For this review, use the dimensioned drawing (mm, ordinates from the lowest corner) and the shaded views. Coordinates: 2 decimals unless noted, no trailing zeros. Loops run counter-clockwise (first coordinate to the right, second up) from the corner with the lowest first, then second, coordinate; pieces in that order, holes last. Notation, with made-up numbers: (82.5, 12.25) - (117.5, 12.25) arc R17 ccw to (117.5, 21.25) - close; hole circle Ø6 at (29.5, -4). An arc over 180 degrees is marked (long way). One line per item, written item: value. Start each with the question number.
1. Insertion check: P1, Ø1.5, axis at y = 11, z = 1, coming from the -X side; P2, Ø1.5, axis at y = 11, z = 2, coming from the +X side; P3, Ø1.5, axis at x = 12.5, z = 1, coming from the +Y side. Each pin has a flat end and moves straight along its axis. Give the tip position at first contact, or say it passes through.
2. We need section D-D, the plane x = 27.5. Give the boundary of the cut face in (y, z).
3. To check wall thickness, follow line 1 (Y direction, x = 13.5, z = 1.5) (1 decimal); line 2 (Y direction, x = 33, z = 1.6) (1 decimal); line 3 (Y direction, x = 17, z = 2.15) (1 decimal). State the ranges of each line that lie inside material, in increasing order.
4. Mouldability with a two-part tool opening along X and no side actions: class the marked faces 1, 2, 3 and 4 as +X half, -X half, draft (parallel to the pull), parting line (faces both ways), or undercut.
5. We need section C-C, the plane z = 1.8. Give the boundary of the cut face in (x, y) (1 decimal), then the cut area to 3 significant figures.
6. We need section A-A, the plane x = 14. Give the boundary of the cut face in (y, z).
7. We need section B-B, the plane y = 12. Give the boundary of the cut face in (x, z).
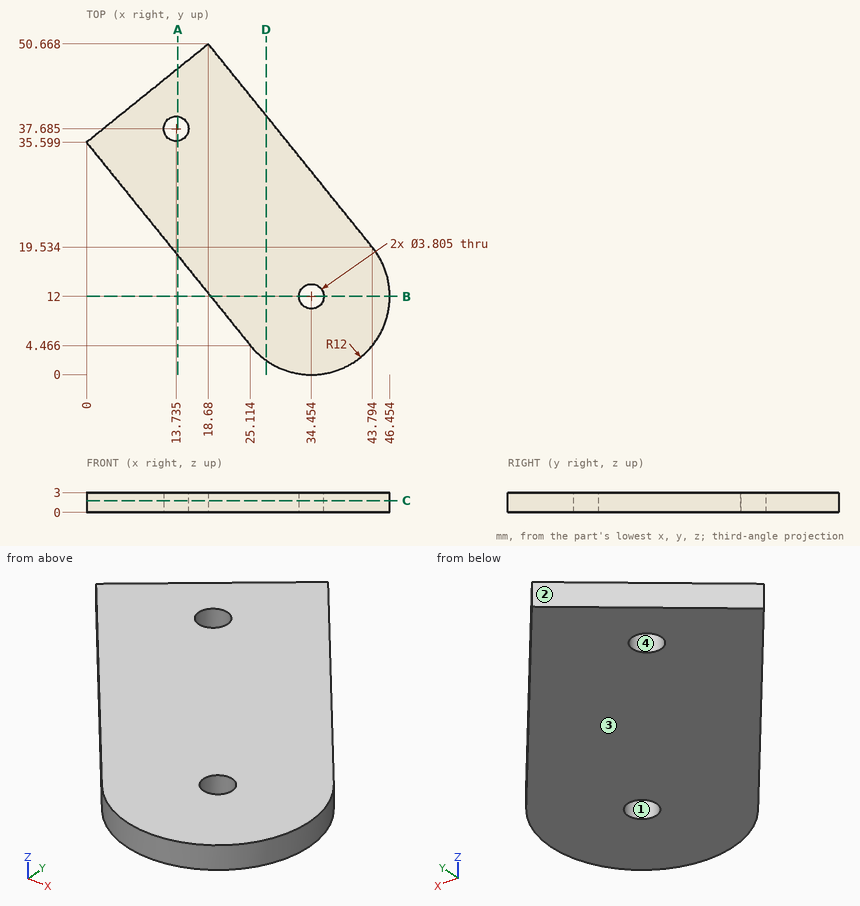
Findings below:
1. P1: x = 19.24
1. P2: x = 46.45
1. P3: y = 46.29
2. outline: (2.22, 0) - (39.73, 0) - (39.73, 3) - (2.22, 3) - close
3. line 1: 18.9 to 35.8, 39.6 to 46.5
3. line 2: 0.1 to 10.8, 13.2 to 32.9
3. line 3: 14.5 to 49.3
4. face 1: undercut
4. face 2: -X half
4. face 3: draft
4. face 4: undercut
5. outline: (0, 35.6) - (25.1, 4.5) arc R12 ccw to (43.8, 19.5) - (18.7, 50.7) - close; hole circle Ø3.8 at (13.7, 37.7); hole circle Ø3.8 at (34.5, 12)
5. area: 1,160 mm2
6. outline: (18.24, 0) - (35.8, 0) - (35.8, 3) - (18.24, 3) - close; (39.57, 0) - (46.89, 0) - (46.89, 3) - (39.57, 3) - close
7. outline: (19.04, 0) - (32.55, 0) - (32.55, 3) - (19.04, 3) - close; (36.36, 0) - (46.45, 0) - (46.45, 3) - (36.36, 3) - close
